```python
from build123d import *

# Parameters (mm, degrees)
SKETCH_1_W          = 93
SKETCH_1_H          = 56
EXTRUDE_1_DEPTH     = 4
SKETCH_2_R          = 1.3
CUT_EXTRUDE_1_DEPTH = 4
SKETCH_3_W          = 5
SKETCH_3_H          = 56
EXTRUDE_2_DEPTH     = 34
SKETCH_4_W          = 103
SKETCH_4_H          = 66
EXTRUDE_3_DEPTH     = 3
CUT_EXTRUDE_2_DEPTH = 21
SKETCH_6_W          = 24
SKETCH_6_H          = 68
EXTRUDE_4_DEPTH     = 5
SKETCH_7_R          = 2.1
CUT_EXTRUDE_3_DEPTH = 5
SKETCH_9_W          = 24
SKETCH_9_H          = 31
SKETCH_9_R          = 1.8
CUT_EXTRUDE_5_DEPTH = 2
SKETCH_10_W         = 20
SKETCH_10_H         = 10
CUT_EXTRUDE_6_DEPTH = 10


with BuildPart() as part:
    # 草圖1 → 填料-伸長1 (new body)
    with BuildSketch(Plane(origin=(0, 0, 0), x_dir=(1, 0, 0), z_dir=(0, 1, 0))):
        with Locations((46.5, 28)):
            Rectangle(SKETCH_1_W, SKETCH_1_H)
    extrude(amount=EXTRUDE_1_DEPTH)

    # 草圖2 → 除料-伸長1 (cut)
    with BuildSketch(Plane(origin=(0, 4, 0), x_dir=(1, 0, 0), z_dir=(0, 1, 0))):
        with Locations(Location((90.5, 53.5, 0), (0, 0, 270))):
            Circle(SKETCH_2_R)
        with Locations(Location((90.5, 2.5, 0), (0, 0, 270))):
            Circle(SKETCH_2_R)
        with Locations(Location((2.5, 53.5, 0), (0, 0, 270))):
            Circle(SKETCH_2_R)
        with Locations(Location((2.5, 2.5, 0), (0, 0, 270))):
            Circle(SKETCH_2_R)
        with Locations(Location((82.5, 2.5, 0), (0, 0, 270))):
            Circle(SKETCH_2_R)
        with Locations(Location((82.5, 53.5, 0), (0, 0, 270))):
            Circle(SKETCH_2_R)
    extrude(amount=-CUT_EXTRUDE_1_DEPTH, mode=Mode.SUBTRACT)

    # 草圖3 → 填料-伸長2 (add)
    with BuildSketch(Plane(origin=(0, 4, 0), x_dir=(1, 0, 0), z_dir=(0, 1, 0))):
        with Locations((-2.5, 28)):
            Rectangle(SKETCH_3_W, SKETCH_3_H)
        Polygon((93, 56), (98, 56), (98, 61), (-5, 61), (-5, 56), (0, 56), align=None)
        with Locations((95.5, 28)):
            Rectangle(SKETCH_3_W, SKETCH_3_H)
        Polygon((98, 0), (98, -5), (-5, -5), (-5, 0), (0, 0), (93, 0), align=None)
    extrude(amount=-EXTRUDE_2_DEPTH)

    # 草圖4 → 填料-伸長3 (add)
    with BuildSketch(Plane(origin=(0, -30, 0), x_dir=(-1, 0, 0), z_dir=(0, -1, 0))):
        with Locations((-46.5, 28)):
            Rectangle(SKETCH_4_W, SKETCH_4_H)
    extrude(amount=EXTRUDE_3_DEPTH)

    # 草圖5 → 除料-伸長2 (cut)
    with BuildSketch(Plane(origin=(0, 4, 0), x_dir=(1, 0, 0), z_dir=(0, 1, 0))):
        Polygon((2.5, 51.5), (5, 51.5), (5, 53.5), (17, 53.5), (17, 51.5), (90.5, 51.5), (90.5, 4.5), (2.5, 4.5), (2.5, 40), (0.5, 40), (0.5, 49.733475986), (2.5, 49.733475986), align=None)
    extrude(amount=-CUT_EXTRUDE_2_DEPTH, mode=Mode.SUBTRACT)

    # 草圖6 → 填料-伸長4 (add)
    with BuildSketch(Plane.XY.offset(5)):
        with Locations((46.5, -30)):
            Rectangle(SKETCH_6_W, SKETCH_6_H)
    extrude(amount=-EXTRUDE_4_DEPTH)

    # 草圖7 → 除料-伸長3 (cut)
    with BuildSketch(Plane.XY.offset(5)):
        with Locations((38.5, -40.5)):
            Circle(SKETCH_7_R)
        with Locations((38.5, -48.5)):
            Circle(SKETCH_7_R)
        with Locations((38.5, -56.5)):
            Circle(SKETCH_7_R)
        with Locations((46.5, -40.5)):
            Circle(SKETCH_7_R)
        with Locations((46.5, -48.5)):
            Circle(SKETCH_7_R)
        with Locations((46.5, -56.5)):
            Circle(SKETCH_7_R)
        with Locations((54.5, -40.5)):
            Circle(SKETCH_7_R)
        with Locations((54.5, -48.5)):
            Circle(SKETCH_7_R)
        with Locations((54.5, -56.5)):
            Circle(SKETCH_7_R)
    extrude(amount=-CUT_EXTRUDE_3_DEPTH, mode=Mode.SUBTRACT)

    # 草圖9 → 除料-伸長5 (cut)
    with BuildSketch(Plane(origin=(0, 0, 0), x_dir=(-1, 0, 0), z_dir=(0, 0, -1))):
        with Locations((-46.5, -48.5)):
            Rectangle(SKETCH_9_W, SKETCH_9_H)
        with Locations((-54.5, -40.5)):
            Circle(SKETCH_9_R, mode=Mode.SUBTRACT)
        with Locations((-46.5, -40.5)):
            Circle(SKETCH_9_R, mode=Mode.SUBTRACT)
        with Locations((-38.5, -40.5)):
            Circle(SKETCH_9_R, mode=Mode.SUBTRACT)
        with Locations((-38.5, -48.5)):
            Circle(SKETCH_9_R, mode=Mode.SUBTRACT)
        with Locations((-46.5, -48.5)):
            Circle(SKETCH_9_R, mode=Mode.SUBTRACT)
        with Locations((-54.5, -48.5)):
            Circle(SKETCH_9_R, mode=Mode.SUBTRACT)
        with Locations((-54.5, -56.5)):
            Circle(SKETCH_9_R, mode=Mode.SUBTRACT)
        with Locations((-46.5, -56.5)):
            Circle(SKETCH_9_R, mode=Mode.SUBTRACT)
        with Locations((-38.5, -56.5)):
            Circle(SKETCH_9_R, mode=Mode.SUBTRACT)
    extrude(amount=-CUT_EXTRUDE_5_DEPTH, mode=Mode.SUBTRACT)

    # 草圖10 → 除料-伸長6 (cut)
    with BuildSketch(Plane.XY.offset(5)):
        with Locations((80, -2.85)):
            Rectangle(SKETCH_10_W, SKETCH_10_H)
    extrude(amount=-CUT_EXTRUDE_6_DEPTH, mode=Mode.SUBTRACT)


solid = part.part
```
For this review, take the finished solid that the model builds, in its own axes (mm). A direction names the side the tool comes from. Give positions to 0.01 mm unless a question says otherwise; leave off trailing zeros. Order: outer loops, then holes, each group sorted by start corner. A loop starts at its lowest first (then second) coordinate and runs counter-clockwise, first axis right, second up.
1) Wall thickness on line 1 (X direction, y = 0.95, z = -2.5); line 2 (X direction, y = 2.2, z = -2.5); line 3 (Z direction, x = 55.5, y = -18.5): over which ranges is each line inside the solid? List them lowest first.
2) Take a section at D-D (y = -56.5). Give the boundary of the cut face in (x, z).
3) Take a section at B-B (z = -2.5). Give the boundary of the cut face in (x, y), then the cut area to 3 significant figures.
4) Take a section at C-C (x = 38.5). Give the boundary of the cut face in (y, z).
5) Insertion check: pin 1 (3.5 mm diameter, centred on x = 2.5, z = -2.5, fed in from -Y); pin 2 (1 mm diameter, centred on x = 70.5, z = -28, fed in from +Y); pin 3 (3.5 mm diameter, centred on x = 46.5, y = -56.5, fed in from -Z); pin 4 (5.5 mm diameter, centred on x = 38.5, y = -40.5, fed in from -Z). Each pin has a flat end and moves straight along its axis. Give the tip position at first contact, or say it passes through.
6) Take a section at A-A (x = 80). Give the boundary of the cut face in (y, z).
7) The part is to be moulded in two halves that separate along Y. For faces 1 (the face through (47.469, -42.363, 3.521)), 2 (the face through (53, 2, -51.5)), 3 (the face through (46, -64, 4)), say which applies: released by +Y, released by -Y, zero draft, split by the parting line, or undercut.
8) For faces 4 (the face through (2.89, 2.03, -1.26)), 5 (the face through (70, -2, 1)), 6 (the face through (0, -15, -28)), list the 3-axis set-ups (+Z, -Z, +X, -X, +Y, -Y) from which the entire face can be reached by the end or side of a thin tool; tool diameter is ignored.
Derived:
1. line 1: x = -5 to 1.2, 3.8 to 70, 91.8 to 98
1. line 2: x = -5 to 1.2, 3.8 to 81.2, 83.8 to 89.2, 91.8 to 98
1. line 3: z = -61 to -56, 0 to 5
2. outline: (34.5, 2) - (36.4, 2) - (36.4, 5) - (34.5, 5) - close; (40.6, 2) - (44.4, 2) - (44.4, 5) - (40.6, 5) - close; (48.6, 2) - (52.4, 2) - (52.4, 5) - (48.6, 5) - close; (56.6, 2) - (58.5, 2) - (58.5, 5) - (56.6, 5) - close
3. outline: (-5, -33) - (98, -33) - (98, 4) - (91.8, 4) - (91.8, 0) - (93, 0) - (93, -30) - (0, -30) - (0, 0) - (1.2, 0) - (1.2, 4) - (-5, 4) - close; (3.8, 0) - (70, 0) - (70, 2.15) - (81.2, 2.15) - (81.2, 4) - (3.8, 4) - close; (83.8, 2.15) - (89.2, 2.15) - (89.2, 4) - (83.8, 4) - close
3. area: 954 mm2
4. outline: (-64, 2) - (-58.6, 2) - (-58.6, 5) - (-64, 5) - close; (-54.4, 2) - (-50.6, 2) - (-50.6, 5) - (-54.4, 5) - close; (-46.4, 2) - (-42.6, 2) - (-42.6, 5) - (-46.4, 5) - close; (-38.4, 2) - (-33, 2) - (-33, -61) - (4, -61) - (4, -51.5) - (0, -51.5) - (0, -56) - (-30, -56) - (-30, 0) - (0, 0) - (0, -4.5) - (4, -4.5) - (4, 5) - (-38.4, 5) - close
5. pin 1: stops at y = -33
5. pin 2: stops at y = -30
5. pin 3: passes through
5. pin 4: stops at z = 2
6. outline: (-33, -61) - (4, -61) - (4, -51.5) - (0, -51.5) - (0, -56) - (-30, -56) - (-30, 0) - (-7.85, 0) - (-7.85, 5) - (-33, 5) - close; (2.15, -4.5) - (4, -4.5) - (4, 5) - (2.15, 5) - close
7. face 1: undercut
7. face 2: zero draft
7. face 3: released by -Y
8. face 4: +Y
8. face 5: +Z
8. face 6: none
